from build123d import *

# Parameters (mm, degrees)
SKETCH1_W           = 120
SKETCH1_H           = 100
BOSS_EXTRUDE1_DEPTH = 75
SKETCH2_W           = 100
SKETCH2_H           = 100
CUT_EXTRUDE1_DEPTH  = 40
SKETCH6_W           = 15.5
SKETCH6_H           = 15.5
CUT_EXTRUDE4_DEPTH  = 100
SKETCH8_W           = 19.1
SKETCH8_H           = 10
CUT_EXTRUDE5_DEPTH  = 100
SKETCH6_3_R         = 5.95
CUT_EXTRUDE6_DEPTH  = 111


with BuildPart() as part:
    # Sketch1 → Boss-Extrude1 (new body)
    with BuildSketch(Plane(origin=(0, 0, 0), x_dir=(1, 0, 0), z_dir=(0, 1, 0))):
        with Locations((-3.53539823, -7.581858407)):
            Rectangle(SKETCH1_W, SKETCH1_H)
    extrude(amount=BOSS_EXTRUDE1_DEPTH)

    # Sketch2 → Cut-Extrude1 (cut)
    with BuildSketch(Plane(origin=(0, 75, 0), x_dir=(1, 0, 0), z_dir=(0, 1, 0))):
        with Locations((-13.53539823, -7.581858407)):
            Rectangle(SKETCH2_W, SKETCH2_H)
    extrude(amount=-CUT_EXTRUDE1_DEPTH, mode=Mode.SUBTRACT)

    # Sketch6 → Cut-Extrude4 (cut)
    with BuildSketch(Plane.ZY.offset(63.53539823)):
        with Locations((-27.068141593, 27.25)):
            Rectangle(SKETCH6_W, SKETCH6_H)
        with Locations((-3.968141593, 27.25)):
            Rectangle(SKETCH6_W, SKETCH6_H)
        with Locations((19.131858407, 27.25)):
            Rectangle(SKETCH6_W, SKETCH6_H)
        with Locations((42.231858407, 27.25)):
            Rectangle(SKETCH6_W, SKETCH6_H)
    extrude(amount=-CUT_EXTRUDE4_DEPTH, mode=Mode.SUBTRACT)

    # Sketch8 → Cut-Extrude5 (cut)
    with BuildSketch(Plane.ZY.offset(63.53539823)):
        with Locations((-27.068141593, 14.5)):
            Rectangle(SKETCH8_W, SKETCH8_H)
        with Locations((-3.968141593, 14.5)):
            Rectangle(SKETCH8_W, SKETCH8_H)
        with Locations((42.231858407, 14.5)):
            Rectangle(SKETCH8_W, SKETCH8_H)
        with Locations((19.131858407, 14.5)):
            Rectangle(SKETCH8_W, SKETCH8_H)
    extrude(amount=-CUT_EXTRUDE5_DEPTH, mode=Mode.SUBTRACT)

    # Sketch6<3> → Cut-Extrude6 (cut)
    with BuildSketch(Plane.ZY.offset(63.53539823)):
        with Locations((-27.068141593, 27.25)):
            Circle(SKETCH6_3_R)
        with Locations((-3.968141593, 27.25)):
            Circle(SKETCH6_3_R)
        with Locations((42.231858407, 27.25)):
            Circle(SKETCH6_3_R)
        with Locations((19.131858407, 27.25)):
            Circle(SKETCH6_3_R)
    extrude(amount=-CUT_EXTRUDE6_DEPTH, mode=Mode.SUBTRACT)


solid = part.part
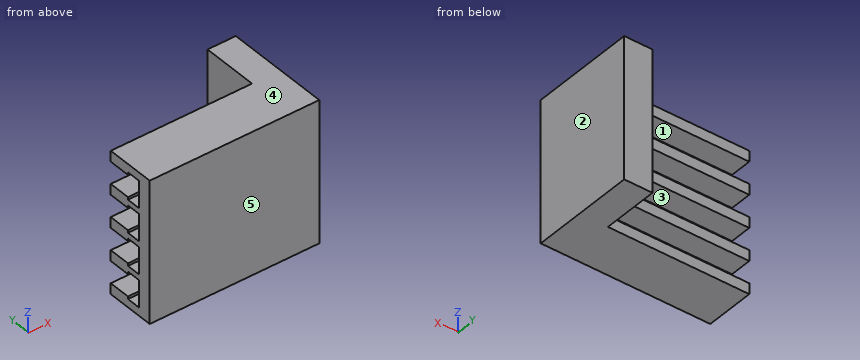
The listing builds one solid part. Answer for the finished solid, in the listing's coordinates (mm). Face numbers are marked on the shaded views. A direction names the side the tool comes from. Round coordinates to 2 decimals unless told otherwise and drop trailing zeros. Write each loop counter-clockwise with the first axis right and the second up, starting at its lowest first coordinate (ties: lowest second). Pieces come first, ordered by that corner, then holes. Notation, with made-up numbers: (89.25, 33) - (118.25, 33) arc R12 ccw to (118.25, 55) - close; hole circle Ø7 at (-33.75, -34.5). An arc over 180 degrees is marked (long way). Use a Markdown table: item, result. Add a question column.
1. Flat-ended cylindrical pins translate along their axes: P1, Ø4, axis at x = -2, z = 8, coming from the +Y side; P2, Ø5, axis at x = 31.5, z = -24.5, coming from the +Y side. Find the tip coordinate at first contact, or state that the pin passes through.
2. The part is cut by section C-C (z = 16.5). Write down the section's boundary in (x, y), and give its area (3 significant figures).
3. For a pull along Z with two mould halves and no side action, classify the marked faces 3, 4 and 5 as +Z half, -Z half, draft (parallel to the pull), parting line (faces both ways), or undercut.
4. A tool of negligible diameter and unlimited length cuts with its end or side. For the marked faces 1 and 2, from which of +Z, -Z, +X, -X, +Y, -Y can it reach the whole face along a straight path? Write none if from no direction.
5. The part is cut by section B-B (y = 50.5). Write down the section's boundary in (x, z), and give its area (3 significant figures).
6. Consider line 1 (Z direction, x = 12, y = 14.5); line 2 (Z direction, x = 45, y = 27); line 3 (Y direction, x = 14, z = 33). Determine where each line is inside the solid, lowest interval first.
7. The part is cut by section A-A (z = -15.5). Write down the section's boundary in (x, y).
Reported:
| question | item | result |
|---|---|---|
| 1 | P1 | y = 35 |
| 1 | P2 | y = 9.5 |
| 2 | outline | (-63.54, 0) - (56.46, 0) - (56.46, 75) - (36.46, 75) - (36.46, 32.59) - (47.46, 32.59) - (47.46, 21.91) - (36.46, 21.91) - (36.46, 9.5) - (-63.54, 9.5) - close |
| 2 | area | 2,330 mm^2 |
| 3 | face 3 | undercut |
| 3 | face 4 | +Z half |
| 3 | face 5 | draft |
| 4 | face 1 | -X, +Y |
| 4 | face 2 | +Z, -Z, +X, +Y, -Y |
| 5 | outline | (36.46, -42.42) - (56.46, -42.42) - (56.46, 57.58) - (36.46, 57.58) - close |
| 5 | area | 2,000 mm^2 |
| 6 | line 1 | -42.42 to -36.62, -17.52 to -13.52, 5.58 to 9.58, 28.68 to 32.68, 51.78 to 57.58 |
| 6 | line 2 | -42.42 to -33.01, -21.12 to -9.91, 1.98 to 13.19, 25.08 to 36.29, 48.18 to 57.58 |
| 6 | line 3 | 0 to 9.5, 19.5 to 35 |
| 7 | outline | (-63.54, 0) - (56.46, 0) - (56.46, 75) - (36.46, 75) - (36.46, 35) - (-63.54, 35) - close |
